from build123d import *

# Parameters (mm, degrees)
SKETCH1_W           = 75
SKETCH1_H           = 35
BOSS_EXTRUDE1_DEPTH = 4
SKETCH2_W           = 4
SKETCH2_H           = 35
BOSS_EXTRUDE2_DEPTH = 40
SKETCH3_R           = 5
CUT_EXTRUDE1_DEPTH  = 62.664414373
FILLET1_R           = 17.5


with BuildPart() as part:
    # Sketch1 → Boss-Extrude1 (new body)
    with BuildSketch(Plane(origin=(0, 0, 0), x_dir=(1, 0, 0), z_dir=(0, 1, 0))):
        Rectangle(SKETCH1_W, SKETCH1_H)
    extrude(amount=BOSS_EXTRUDE1_DEPTH)

    # Sketch2 → Boss-Extrude2 (add)
    with BuildSketch(Plane(origin=(0, 4, 0), x_dir=(1, 0, 0), z_dir=(0, 1, 0))):
        Rectangle(SKETCH2_W, SKETCH2_H)
    extrude(amount=BOSS_EXTRUDE2_DEPTH)

    # Sketch3 → Cut-Extrude1 (cut, through all)
    with BuildSketch(Plane(origin=(2, 0, 0), x_dir=(0, 0, -1), z_dir=(1, 0, 0))):
        with Locations((0, 29)):
            Circle(SKETCH3_R)
    extrude(amount=-CUT_EXTRUDE1_DEPTH, mode=Mode.SUBTRACT)

    # Fillet1
    fillet1_edges = [part.edges().sort_by_distance(p)[0] for p in [
        (0, 44, -17.5),
        (0, 44, 17.5),
    ]]
    fillet(fillet1_edges, radius=FILLET1_R - 0.0001)  # a hair under: the kernel refuses the full size


solid = part.part
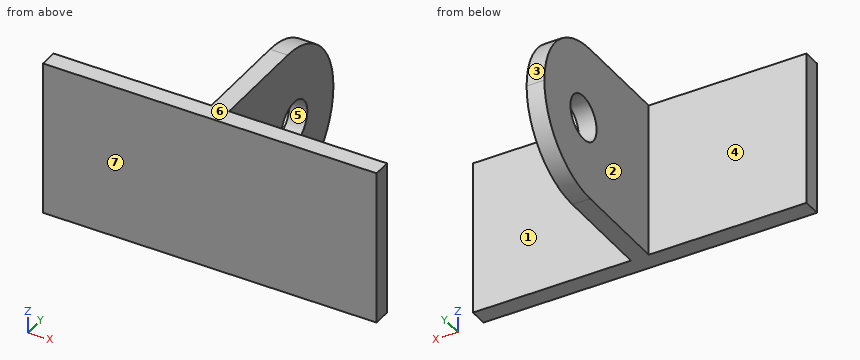
Read the model definition and answer for the solid it produces. Units are mm, in the model's axes. Face numbers are marked on the shaded views. A direction names the side the tool comes from. Round coordinates to 2 decimals unless told otherwise and drop trailing zeros. Order: outer loops, then holes, each group sorted by start corner. A loop starts at its lowest first (then second) coordinate and runs counter-clockwise, first axis right, second up. Notation, with made-up numbers: (89.5, -9.5) - (121.5, -9.5) arc R16 cw to (121.5, 8.5) - close; hole circle Ø1 at (74, -28.5). An arc over 180 degrees is marked (long way). Use one line per item in the form item = value. Start each with the question number.
(1) Determine the mould class of the marked faces 4, 5, 6 and 7 for opening direction Y: +Y half, -Y half, draft (parallel to the pull), parting line (faces both ways), or undercut.
(2) For the marked faces 1, 2 and 3, determine the directions among +Z, -Z, +X, -X, +Y, -Y from which every point of the face is accessible in a straight line to the end or side of a thin tool.
(3) Flat-ended cylindrical pins translate along their axes: pin 1 Ø1.5 at (x, z) = (25, -1.5) entering from +Y; pin 2 Ø4 at (y, z) = (20.5, 9.5) entering from +X; pin 3 Ø12 at (y, z) = (38, -3) entering from -X. Find the tip coordinate at first contact, or state that the pin passes through.
(4) The part is cut by section A-A (y = 29). Give the vertices of the cut face in (x, z), then the cut area to 3 significant figures.
(5) The part is cut by section B-B (x = 31). Give the vertices of the cut face in (y, z), then the cut area to 3 significant figures.
(6) Find the intervals of material crossed by line 1 along Y through (x, z) = (1, 0); line 2 along X through (y, z) = (19.5, 7); line 3 along Y through (x, z) = (-17, 11.5), in increasing order. Write a range as from..to.
(7) The part is cut by section D-D (y = 19.5). Give the vertices of the cut face in (x, z), then the cut area to 3 significant figures.
(8) The part is cut by section C-C (z = -6). Give the vertices of the cut face in (x, y), then the cut area to 3 significant figures.
Checked values:
q1.face_4 = +Y half
q1.face_5 = undercut
q1.face_6 = draft
q1.face_7 = -Y half
q2.face_1 = +Z, -Z, +X, +Y
q2.face_2 = +Z, -Z, -X, +Y
q2.face_3 = +Z, +X, -X, +Y
q3.pin_1 = 4
q3.pin_2 = 2
q3.pin_3 = -2
q4.outline = (-2, -17.32) - (2, -17.32) - (2, -5) - (-2, -5) - close; (-2, 5) - (2, 5) - (2, 17.32) - (-2, 17.32) - close
q4.area = 98.6 mm^2
q5.outline = (0, -17.5) - (4, -17.5) - (4, 17.5) - (0, 17.5) - close
q5.area = 140 mm^2
q6.line_1 = 0..24, 34..44
q6.line_2 = -2..2
q6.line_3 = 0..4
q7.outline = (-2, -17.5) - (2, -17.5) - (2, 17.5) - (-2, 17.5) - close
q7.area = 140 mm^2
q8.outline = (-37.5, 0) - (37.5, 0) - (37.5, 4) - (2, 4) - (2, 42.94) - (-2, 42.94) - (-2, 4) - (-37.5, 4) - close
q8.area = 456 mm^2
